Work out the finished part from the listing and answer in its coordinate system (mm). Face numbers are marked on the shaded views. A direction names the side the tool comes from. Round coordinates to 2 decimals unless told otherwise and drop trailing zeros. Write each loop counter-clockwise with the first axis right and the second up, starting at its lowest first coordinate (ties: lowest second). Pieces come first, ordered by that corner, then holes. Notation, with made-up numbers: M 14,42 L 33,42 A25 ccw 33,66 Z; hole C 52.5,6 d10. An arc over 180 degrees is marked long. Answer in a Markdown table with one row per item.
```python
from build123d import *

# Parameters (mm, degrees)
F0_W          = 2
F0_H          = 14.5
F0_W_2        = 3
F0_H_2        = 3
F0_W_3        = 29
F0_H_3        = 2
F1_DEPTH      = 22
F2_DEPTH      = 28
F2_DEPTH_BACK = 5
F3_R          = 1.75
F4_DEPTH      = 5
F5_START      = -1
F5_DEPTH      = 4
F6_SIZE2      = 3
F6_SIZE       = 6


# Not quite as in the source:
# - a feature names something its author has since deleted; it is built from what else it names


with BuildPart() as f1:
    # F0 (on Right) → F1 (new body)
    with BuildSketch(Plane.YZ):
        Polygon((-20.25, 5), (-20.25, 0), (-17.25, 0), (17.25, 0), (20.25, 0), (20.25, 5), (18.25, 5), align=None)
        with Locations((19.25, 12.25)):
            Rectangle(F0_W, F0_H)
        with Locations((-18.75, -1.5)):
            Rectangle(F0_W_2, F0_H_2)
        with Locations((18.75, -1.5)):
            Rectangle(F0_W_2, F0_H_2)
        with Locations((3.75, 20.5)):
            Rectangle(F0_W_3, F0_H_3)
        with Locations((19.25, 20.5)):
            Rectangle(F0_W, F0_H_3)
        Polygon((-10.75, 17.5), (-10.75, 19.5), (-10.75, 21.5), (-12.75, 21.5), (-12.75, 17.5), align=None)
    extrude(amount=F1_DEPTH)

    # F0 (on Right) → F2 (join, two sides)
    with BuildSketch(Plane.YZ) as f2_sk:
        Polygon((-20.25, 5), (-20.25, 0), (-17.25, 0), (17.25, 0), (20.25, 0), (20.25, 5), (18.25, 5), align=None)
    extrude(amount=F2_DEPTH)
    extrude(f2_sk.sketch, amount=-F2_DEPTH_BACK)

    # F3 (on face) → F4 (cut, through all)
    with BuildSketch(Plane(origin=(0, 0, 0), x_dir=(1, 0, 0), z_dir=(0, 0, -1))):
        with Locations((11.5, 10)):
            Circle(F3_R)
        with Locations((11.5, -10)):
            Circle(F3_R)
    extrude(amount=-F4_DEPTH, mode=Mode.SUBTRACT)

    # F3 (on face) → F5 (cut)
    with BuildSketch(Plane(origin=(0, 0, 0), x_dir=(1, 0, 0), z_dir=(0, 0, -1)).offset(F5_START)):
        Polygon((8.75, -8.4122867597), (8.75, -11.5877132403), (11.5, -13.1754264805), (14.25, -11.5877132403), (14.25, -8.4122867597), (11.5, -6.8245735195), align=None)
        with Locations((11.5, -10)):
            Circle(F3_R, mode=Mode.SUBTRACT)
        Polygon((8.75, 11.5877132403), (8.75, 8.4122867597), (11.5, 6.8245735195), (14.25, 8.4122867597), (14.25, 11.5877132403), (11.5, 13.1754264805), align=None)
        with Locations((11.5, 10)):
            Circle(F3_R, mode=Mode.SUBTRACT)
    extrude(amount=-F5_DEPTH, mode=Mode.SUBTRACT)

    # F6
    f6_edges = [f1.edges().sort_by_distance(p)[0] for p in [
        (28, 0, 5),
        (11.5, -20.25, 5),
        (-5, 0, 5),
    ]]
    f6_side = f1.faces().sort_by_distance((11.51774, -0.683006, 5))[0]
    chamfer(f6_edges, length=F6_SIZE, length2=F6_SIZE2, reference=f6_side)


solid = f1.part
```
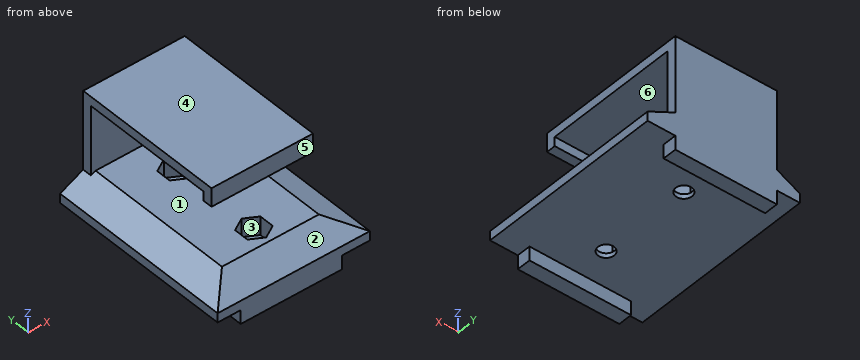
1. The part is cut by section A-A (y = 4.5). Determine the outline of the cut face in (x, z).
Calculated:
| item | result |
|---|---|
| outline | M -5,0 L 28,0 L 28,2 L 22,5 L 1,5 L -5,2 Z; M 0,19.5 L 22,19.5 L 22,21.5 L 0,21.5 Z |
2. A tool of negligible diameter and unlimited length cuts with its end or side. For the marked faces 1, 2 and 3, from which of +Z, -Z, +X, -X, +Y, -Y can it reach the whole face along a straight path? Write none if from no direction.
Calculated:
| item | result |
|---|---|
| face 1 | +X, -X, -Y |
| face 2 | +Z, +X, -X, -Y |
| face 3 | none |
3. The part is cut by section B-B (y = 10). Determine the outline of the cut face in (x, z).
Calculated:
| item | result |
|---|---|
| outline | M -5,0 L 9.75,0 L 9.75,1 L 8.75,1 L 8.75,5 L 1,5 L -5,2 Z; M 0,19.5 L 22,19.5 L 22,21.5 L 0,21.5 Z; M 13.25,0 L 28,0 L 28,2 L 22,5 L 14.25,5 L 14.25,1 L 13.25,1 Z |
4. Consider line 1 along Y through (x, z) = (11.5, 0.6); line 2 along Z through (x, y) = (14.5, 7.5); line 3 along Y through (x, z) = (9.5, 3.25). Determine where each line is inside the solid, lowest interval first. Write a range as from..to.
Calculated:
| item | result |
|---|---|
| line 1 | y = -20.25..-11.75, -8.25..8.25, 11.75..20.25 |
| line 2 | z = 0..5, 19.5..21.5 |
| line 3 | y = -17.75..-12.02, -7.98..7.98, 12.02..20.25 |
5. Determine the mould class of the marked faces 4, 5 and 6 for opening direction Y: released by +Y, released by -Y, zero draft, split by the parting line, or undercut.
Calculated:
| item | result |
|---|---|
| face 4 | zero draft |
| face 5 | released by -Y |
| face 6 | undercut |
6. Given pin 1 (1.5 mm diameter, centred on y = -19.5, z = -1.5, fed in from +X); pin 2 (1 mm diameter, centred on x = 1.5, z = 4.5, fed in from -Y); pin 3 (3 mm diameter, centred on x = 17, y = 12, fed in from -Z); pin 4 (2.5 mm diameter, centred on y = -9, z = 3, fed in from -X), each flat-ended and moving along its own axis, determine where each tip first touches the part or whether it passes through.
Calculated:
| item | result |
|---|---|
| pin 1 | stops at x = 22 |
| pin 2 | stops at y = -16.25 |
| pin 3 | stops at z = 0 |
| pin 4 | stops at x = -5 |
7. The part is cut by section D-D (x = 3.5). Determine the outline of the cut face in (y, z).
Calculated:
| item | result |
|---|---|
| outline | M -20.25,-3 L -17.25,-3 L -17.25,0 L 17.25,0 L 17.25,-3 L 20.25,-3 L 20.25,21.5 L -12.75,21.5 L -12.75,17.5 L -10.75,17.5 L -10.75,19.5 L 18.25,19.5 L 18.25,5 L -14.25,5 L -20.25,2 Z |
8. The part is cut by section C-C (x = 11). Count the separate pieces of the cut face and the enclosed holes in it, plus the area to 3 significant figures.
Calculated:
| item | result |
|---|---|
| separate pieces | 3 |
| enclosed holes | 0 |
| area | 258 mm² |
